Geometry check sheet. Reference: the model listing, model coordinates, mm. A direction names the side the tool comes from. Give positions to 0.01 mm unless a question says otherwise; leave off trailing zeros. Order: outer loops, then holes, each group sorted by start corner. A loop starts at its lowest first (then second) coordinate and runs counter-clockwise, first axis right, second up. Notation, with made-up numbers: M -5.5,80 L 8.5,80 A12 ccw 8.5,87 Z; hole C -13,82.5 d10. An arc over 180 degrees is marked long. Use CSV: the item, a comma, the result in double quotes. Start each with the question number.
from build123d import *

# Parameters (mm, degrees)
BOSS_EXTRUDE1_DEPTH     = 35
BOSS_EXTRUDE1_2_DEPTH   = 35
SKETCH4_W               = 56
SKETCH4_H               = 126
BOSS_EXTRUDE2_DEPTH     = 12
SKETCH5_W               = 52
SKETCH5_H               = 122
CUT_EXTRUDE1_DEPTH      = 10
CUT_EXTRUDE2_DEPTH      = 113.915897906
CUT_EXTRUDE2_DEPTH_BACK = 113.915897906
SKETCH6_W               = 40
SKETCH6_H               = 50
SKETCH6_W_2             = 7
SKETCH6_H_2             = 26


with BuildPart() as part:
    # Sketch3 → Boss-Extrude1 (new, symmetric)
    with BuildSketch(Plane(origin=(0, 0, 0), x_dir=(0, 0, -1), z_dir=(1, 0, 0))):
        Polygon((24, 0), (24, -50), (27, -50), (27, -35), (32, -35), (32, 0), align=None)
    extrude(amount=BOSS_EXTRUDE1_DEPTH, both=True)



with BuildPart() as body_2:
    # Sketch3 → Boss-Extrude1 2 (new, symmetric)
    with BuildSketch(Plane(origin=(0, 0, 0), x_dir=(0, 0, -1), z_dir=(1, 0, 0))):
        Polygon((-32, 0), (-24, 0), (-24, -50), (-27, -50), (-27, -35), (-32, -35), align=None)
    extrude(amount=BOSS_EXTRUDE1_2_DEPTH, both=True)


with BuildPart() as part_1:
    add(part.part)

    add(body_2.part)  # Boss-Extrude2 merges body 2
    # Sketch4 → Boss-Extrude2 (add)
    with BuildSketch(Plane(origin=(0, 0, 0), x_dir=(1, 0, 0), z_dir=(0, 1, 0))):
        Rectangle(SKETCH4_W, SKETCH4_H)
    extrude(amount=BOSS_EXTRUDE2_DEPTH)

    # Sketch5 → Cut-Extrude1 (cut)
    with BuildSketch(Plane(origin=(0, 12, 0), x_dir=(1, 0, 0), z_dir=(0, 1, 0))):
        Rectangle(SKETCH5_W, SKETCH5_H)
    extrude(amount=-CUT_EXTRUDE1_DEPTH, mode=Mode.SUBTRACT)

    # Sketch6 → Cut-Extrude2 (cut, two sides: drawn at the far end of the back side and taken through both)
    with BuildSketch(Plane.XY.offset(32).offset(-CUT_EXTRUDE2_DEPTH_BACK)):
        with Locations((0, -25)):
            Rectangle(SKETCH6_W, SKETCH6_H)
        with Locations((-31.5, -13)):
            Rectangle(SKETCH6_W_2, SKETCH6_H_2)
        with Locations((31.5, -13)):
            Rectangle(SKETCH6_W_2, SKETCH6_H_2)
    extrude(amount=CUT_EXTRUDE2_DEPTH + CUT_EXTRUDE2_DEPTH_BACK, mode=Mode.SUBTRACT)


solid = part_1.part
(1) Sectioned sample at C-C on x = 9. Record the cut outline in (y, z), then the cut area to 3 significant figures.
(2) Sectioned sample at A-A on y = -42.5. Record the cut outline in (x, z), then the cut area to 3 significant figures.
(3) Sectioned sample at D-D on y = 6.5. Record the cut outline in (x, z).
(4) Draft check along X on faces 1 (the face through (-20, -20, 28)), 2 (the face through (-35, -35, -26)), 3 (the face through (0, 7, 61)), 4 (the face through (-26, -30, 24)). Enter one of: +X half, -X half, draft (parallel to the pull), parting line (faces both ways), or undercut.
(5) Go/stop test with flat-tipped pins: P1, Ø8, axis at x = -2, z = 5, coming from the +Y side; P2, Ø12, axis at x = 31, y = -10, coming from the -Z side; P3, Ø16.5, axis at x = 24, y = -24, coming from the +Z side. Record where each tip stops, or that it passes through.
(6) Sectioned sample at B-B on z = 28.5. Record the cut outline in (x, y).
(7) Access from +Z, -Z, +X, -X, +Y, -Y to the whole of each face (thin tool, end or side, straight path). Record for faces 5 (the face through (28, -43, 27)), 6 (the face through (28, -35, -29)), 7 (the face through (26, -30, 24)), 8 (the face through (20, -20, 28)).
(8) Thickness scan on line 1 (Z direction, x = -9, y = 5); line 2 (X direction, y = 5.5, z = 12.5); line 3 (Y direction, x = 5.5, z = 24). Record the ranges inside material, lowest first.
Responses:
1,outline,"M 0,-63 L 12,-63 L 12,-61 L 2,-61 L 2,61 L 12,61 L 12,63 L 0,63 Z"
1,area,"292 mm2"
2,outline,"M -35,-27 L -20,-27 L -20,-24 L -35,-24 Z; M -35,24 L -20,24 L -20,27 L -35,27 Z; M 20,-27 L 35,-27 L 35,-24 L 20,-24 Z; M 20,24 L 35,24 L 35,27 L 20,27 Z"
2,area,"180 mm2"
3,outline,"M -28,-63 L 28,-63 L 28,63 L -28,63 Z; hole M -26,-61 L 26,-61 L 26,61 L -26,61 Z"
4,face 1,"undercut"
4,face 2,"-X half"
4,face 3,"undercut"
4,face 4,"draft"
5,P1,"y = 2"
5,P2,"z = -32"
5,P3,"z = 32"
6,outline,"M -35,-35 L -20,-35 L -20,0 L 20,0 L 20,-35 L 35,-35 L 35,-26 L 28,-26 L 28,12 L 26,12 L 26,2 L -26,2 L -26,12 L -28,12 L -28,-26 L -35,-26 Z"
7,face 5,"+Z, +X, -X, -Y"
7,face 6,"-Z, +X, -X, -Y"
7,face 7,"+X, -X, -Y"
7,face 8,"+Z, -Z, -Y"
8,line 1,"-63 to -61, 61 to 63"
8,line 2,"-28 to -26, 26 to 28"
8,line 3,"0 to 2"
